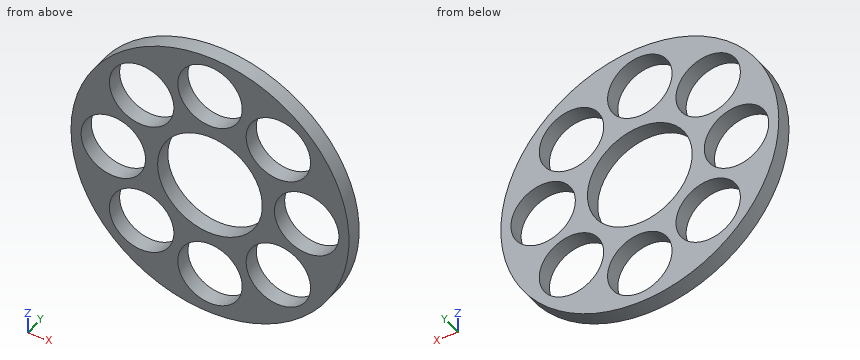
Autodesk Inventor part; units mm, degrees
ref_plane "YZ Plane" through (0, 0, 0) normal (1, 0, 0) x (0, 1, 0)
ref_plane "XZ Plane" through (0, 0, 0) normal (0, 1, 0) x (-1, 0, 0)
ref_plane "XY Plane" through (0, 0, 0) normal (0, 0, 1) x (1, 0, 0)
sketch "Sketch1" plane through (0, 0, 0) normal (0, 1, 0) x (-1, 0, 0)
  line L0 (0, 0) -> (12, 0) construction
  circle A0 centre (12, 0) radius 4
  circle A1 centre (8.4853, 8.4853) radius 4
  circle A2 centre (0, 12) radius 4
  circle A3 centre (-8.4853, 8.4853) radius 4
  circle A4 centre (-12, 0) radius 4
  circle A5 centre (-8.4853, -8.4853) radius 4
  circle A6 centre (0, -12) radius 4
  circle A7 centre (8.4853, -8.4853) radius 4
  circle A8 centre (0, 0) radius 17.25
  circle A9 centre (0, 0) radius 6.5
  dimension "d0" = 12
  dimension "d1" = 8
  dimension "d4" = 360
  dimension "d6" = 34.5
  dimension "d9" = 13
extrude "Extrusion1" add sketch "Sketch1" along normal blind 2
properties part number "tubeholder"
Could you check a few things on this model? Use its own coordinates, in mm. Give positions to 0.01 mm unless a question says otherwise; leave off trailing zeros. Write each loop counter-clockwise with the first axis right and the second up, starting at its lowest first coordinate (ties: lowest second). Pieces come first, ordered by that corner, then holes. Notation, with made-up numbers: (-28, 21) - (-22, 21) arc R27 cw to (-22, 37) - close; hole circle Ø2 at (76.25, 5). An arc over 180 degrees is marked (long way). Use CSV: the item, a comma, the result in double quotes. Start each with the question number.
Item 1: I want a section at C-C, the plane z = -7. Please give me the cut outline in (x, y).
Item 2: I want a section at B-B, the plane z = 12. Please give me the cut outline in (x, y).
Item 3: If I drill on line 1 along Z through (x, y) = (0, 0.7); line 2 along X through (y, z) = (1.4, -11.5); line 3 along Z through (x, y) = (5, 1.25), over which ranges is the centre line in solid material (lowest first)?
Item 4: I want a section at A-A, the plane x = 0. Please give me the cut outline in (y, z), then the cut area to 3 significant figures.
Item 5: I want a section at D-D, the plane y = 1.6. Give the number of separate pieces and of enclosed holes in the cut face, then the cut area to 3 significant figures.
Findings:
1,outline,"(-15.77, 0) - (-12.2, 0) - (-12.2, 2) - (-15.77, 2) - close; (-4.77, 0) - (4.77, 0) - (4.77, 2) - (-4.77, 2) - close; (12.2, 0) - (15.77, 0) - (15.77, 2) - (12.2, 2) - close"
2,outline,"(-12.39, 0) - (-10.39, 0) - (-10.39, 2) - (-12.39, 2) - close; (-6.58, 0) - (-4, 0) - (-4, 2) - (-6.58, 2) - close; (4, 0) - (6.58, 0) - (6.58, 2) - (4, 2) - close; (10.39, 0) - (12.39, 0) - (12.39, 2) - (10.39, 2) - close"
3,line 1,"z = -17.25 to -16, -8 to -6.5, 6.5 to 8, 16 to 17.25"
3,line 2,"x = -12.86 to -11.11, -5.86 to -3.97, 3.97 to 5.86, 11.11 to 12.86"
3,line 3,"z = -16.51 to -10.45, -6.52 to -4.15, 4.15 to 6.52, 10.45 to 16.51"
4,outline,"(0, -17.25) - (2, -17.25) - (2, -16) - (0, -16) - close; (0, -8) - (2, -8) - (2, -6.5) - (0, -6.5) - close; (0, 6.5) - (2, 6.5) - (2, 8) - (0, 8) - close; (0, 16) - (2, 16) - (2, 17.25) - (0, 17.25) - close"
4,area,"11.0 mm2"
5,separate pieces,"1"
5,enclosed holes,"9"
5,area,"400 mm2"
